Autodesk Inventor part; units mm, degrees
ref_plane "YZ Plane" through (0, 0, 0) normal (1, 0, 0) x (0, 1, 0)
ref_plane "XZ Plane" through (0, 0, 0) normal (0, 1, 0) x (-1, 0, 0)
ref_plane "XY Plane" through (0, 0, 0) normal (0, 0, 1) x (1, 0, 0)
sketch "스케치1" plane through (0, 0, 0) normal (0, 1, 0) x (-1, 0, 0)
  circle A0 centre (7.6948, -23.9851) radius 1.45
  circle A1 centre (27.7948, -23.9851) radius 1.45
  line L0 (-2.3552, -20.9851) -> (37.8448, -20.9851)
  line L1 (-2.3552, -20.9851) -> (-2.3552, -26.9851)
  line L2 (37.8448, -26.9851) -> (-2.3552, -26.9851)
  line L3 (37.8448, -20.9851) -> (37.8448, -26.9851)
  circle A2 centre (27.7948, 62.4149) radius 1.45
  circle A3 centre (7.6948, 62.4149) radius 1.45
  line L4 (37.8448, 65.4149) -> (-2.3552, 65.4149)
  line L5 (-2.3552, 65.4149) -> (-2.3552, 59.4149)
  line L6 (37.8448, 59.4149) -> (-2.3552, 59.4149)
  line L7 (37.8448, 65.4149) -> (37.8448, 59.4149)
  line L8 (37.8448, -20.9851) -> (-2.3552, -20.9851)
  line L9 (-2.3552, -20.9851) -> (-2.3552, 59.4149)
  line L10 (-2.3552, 59.4149) -> (37.8448, 59.4149)
  line L11 (37.8448, 59.4149) -> (37.8448, -20.9851)
  point P0 (0, 0)
extrude "돌출1" add sketch "스케치1" along normal blind 6 contours L9 L6 L11 L0
sketch "스케치2" plane through (0, 6, 0) normal (0, 1, 0) x (1, 0, 0)
  line L0 (2.3552, 20.9851) -> (-37.8448, 20.9851)
  line L1 (-37.8448, 20.9851) -> (-37.8448, -59.4149)
  line L2 (-37.8448, -59.4149) -> (2.3552, -59.4149)
  line L3 (2.3552, -59.4149) -> (2.3552, 20.9851)
  line L4 (-47.7448, 30.7851) -> (12.2552, -69.2149) construction
  line L5 (12.2552, 30.7851) -> (-47.7448, -69.2149) construction
  circle A0 centre (-7.6948, -39.3149) radius 1.35
  circle A1 centre (-27.7948, -39.3149) radius 1.35
  circle A2 centre (-7.6948, 0.8851) radius 1.35
  circle A3 centre (-27.7948, 0.8851) radius 1.35
  point P0 (0, 0)
  dimension "d2" = 60
  dimension "d3" = 100
  dimension "d4" = 2.7
  dimension "d5" = 2.7
  dimension "d6" = 2.7
  dimension "d27" = 2.7
extrude "돌출2" cut sketch "스케치2" against normal blind 6 contours A0 | A1 | A2 | A3
sketch "스케치3" plane through (-37.8448, 0, 59.4149) normal (0, 0, 1) x (1, 0, 0)
  line L0 (0, 0) -> (40.2, 0)
  line L1 (40.2, 0) -> (40.2, 6)
  line L2 (0, 6) -> (40.2, 6)
  line L3 (0, 0) -> (0, 6)
  line L4 (0, 6) -> (10.05, 6)
  line L5 (10.05, 6) -> (30.15, 6)
  circle A0 centre (10.05, 3) radius 1.35
  circle A1 centre (30.15, 3) radius 1.35
  point P0 (37.8448, 0)
  dimension "d9" = 40.2
  dimension "d10" = 6
  dimension "d11" = 10.05
  dimension "d12" = 20.1
  dimension "d13" = 2.7
  dimension "d14" = 2.7
extrude "돌출3" cut sketch "스케치3" against normal blind 16 contours A0 | A1
sketch "스케치4" plane through (2.3552, 0, -20.9851) normal (0, 0, -1) x (-1, 0, 0)
  circle A0 centre (30.15, 3) radius 1.35
  line L0 (11.4, 6) -> (11.4, 0)
  circle A1 centre (10.05, 3) radius 1.35
  point P0 (2.3552, 0)
extrude "돌출4" cut sketch "스케치4" against normal blind 16
sketch "스케치5" plane through (0, 6, 0) normal (0, 1, 0) x (1, 0, 0)
  line L0 (-29.1448, 20.9851) -> (-29.1448, 4.9851)
  line L1 (-26.4448, 20.9851) -> (-26.4448, 4.9851)
  line L2 (-29.1448, 4.9851) -> (-26.4448, 4.9851)
  line L3 (-9.0448, 20.9851) -> (-9.0448, 4.9851)
  line L4 (-6.3448, 20.9851) -> (-6.3448, 4.9851)
  line L5 (-9.0448, 4.9851) -> (-6.3448, 4.9851)
  circle A0 centre (-7.6948, 0.8851) radius 1.35
  circle A1 centre (-27.7948, 0.8851) radius 1.35
  circle A2 centre (-7.6948, -39.3149) radius 1.35
  circle A3 centre (-27.7948, -39.3149) radius 1.35
  line L6 (2.3552, 20.9851) -> (-37.8448, 20.9851)
  line L7 (-37.8448, 20.9851) -> (-37.8448, -59.4149)
  line L8 (-37.8448, -59.4149) -> (2.3552, -59.4149)
  line L9 (2.3552, -59.4149) -> (2.3552, 20.9851)
  line L10 (-9.0448, -59.4149) -> (-9.0448, -43.4149)
  line L11 (-29.1448, -59.4149) -> (-29.1448, -43.4149)
  line L12 (-26.4448, -59.4149) -> (-26.4448, -43.4149)
  line L13 (-6.3448, -59.4149) -> (-6.3448, -43.4149)
  line L14 (-30.3948, -52.5149) -> (-25.1948, -52.5149)
  line L15 (-25.1948, -52.5149) -> (-25.1948, -50.3149)
  line L16 (-25.1948, -50.3149) -> (-30.3948, -50.3149)
  line L17 (-30.3948, -50.3149) -> (-30.3948, -52.5149)
  line L18 (-30.3948, -52.5149) -> (-25.1948, -50.3149) construction
  line L19 (-25.1948, -52.5149) -> (-30.3948, -50.3149) construction
  line L20 (-10.2948, -52.5149) -> (-5.0948, -52.5149)
  line L21 (-5.0948, -52.5149) -> (-5.0948, -50.3149)
  line L22 (-5.0948, -50.3149) -> (-10.2948, -50.3149)
  line L23 (-10.2948, -50.3149) -> (-10.2948, -52.5149)
  line L24 (-10.2948, -52.5149) -> (-5.0948, -50.3149) construction
  line L25 (-5.0948, -52.5149) -> (-10.2948, -50.3149) construction
  line L26 (-30.3948, 11.8851) -> (-25.1948, 11.8851)
  line L27 (-25.1948, 11.8851) -> (-25.1948, 14.0851)
  line L28 (-25.1948, 14.0851) -> (-30.3948, 14.0851)
  line L29 (-30.3948, 14.0851) -> (-30.3948, 11.8851)
  line L30 (-30.3948, 11.8851) -> (-25.1948, 14.0851) construction
  line L31 (-25.1948, 11.8851) -> (-30.3948, 14.0851) construction
  line L32 (-10.2948, 11.8851) -> (-5.0948, 11.8851)
  line L33 (-5.0948, 11.8851) -> (-5.0948, 14.0851)
  line L34 (-5.0948, 14.0851) -> (-10.2948, 14.0851)
  line L35 (-10.2948, 14.0851) -> (-10.2948, 11.8851)
  line L36 (-10.2948, 11.8851) -> (-5.0948, 14.0851) construction
  line L37 (-5.0948, 11.8851) -> (-10.2948, 14.0851) construction
  point P0 (0, 0)
  point P1 (-27.7948, -51.4149)
  point P2 (-7.6948, -51.4149)
  point P3 (-27.7948, 12.9851)
  point P4 (-7.6948, 12.9851)
  dimension "d34" = 5.2
  dimension "d35" = 2.2
  dimension "d36" = 5.2
  dimension "d37" = 2.2
  dimension "d38" = 5.2
  dimension "d39" = 2.2
  dimension "d40" = 5.2
  dimension "d41" = 2.2
extrude "돌출5" cut sketch "스케치5" against normal blind 6 contours L28 L1 L26 L0 | L0 L26 L29 L28 | L28 L27 L26 L1 | L34 L4 L32 L3 | L3 L32 L35 L34 | L34 L33 L32 L4 | L14 L17 L16 L11 | L11 L16 L12 L14 | L12 L16 L15 L14 | L20 L23 L22 L10 | L10 L22 L13 L20 | L13 L22 L21 L20
sketch "스케치6" plane through (-37.8448, 0, 59.4149) normal (0, 0, 1) x (1, 0, 0)
  circle A0 centre (30.15, 3) radius 1.35
  circle A1 centre (10.05, 3) radius 1.35
  line L0 (0, 0) -> (40.2, 0)
  line L1 (40.2, 0) -> (40.2, 6)
  line L2 (0, 6) -> (40.2, 6)
  line L3 (0, 0) -> (0, 6)
  line L4 (15.1, 0) -> (25.1, 0)
  line L5 (25.1, 0) -> (25.1, 6)
  line L6 (25.1, 6) -> (15.1, 6)
  line L7 (15.1, 6) -> (15.1, 0)
  line L8 (15.1, 0) -> (25.1, 6) construction
  line L9 (25.1, 0) -> (15.1, 6) construction
  point P0 (37.8448, 0)
  point P1 (20.1, 3)
  dimension "d28" = 10
extrude "돌출6" add sketch "스케치6" along normal blind 6 contours L7 L2 L5 L0
sketch "스케치7" plane through (2.3552, 0, -20.9851) normal (0, 0, -1) x (-1, 0, 0)
  line L0 (15.1, 6) -> (15.1, 0)
  line L1 (25.1, 0) -> (25.1, 6)
  circle A0 centre (30.15, 3) radius 1.35
  circle A1 centre (10.05, 3) radius 1.35
  line L2 (0, 0) -> (40.2, 0)
  line L3 (40.2, 0) -> (40.2, 6)
  line L4 (0, 6) -> (40.2, 6)
  line L5 (0, 0) -> (0, 6)
  point P0 (2.3552, 0)
extrude "돌출7" add sketch "스케치7" along normal blind 6 contours L4 L1 L2 L0
properties part number "feet_holder3" material "PMMA 플라스틱"
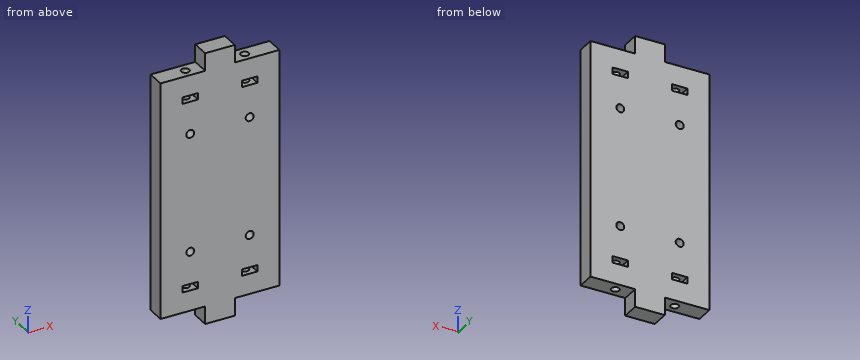
Source: CAD feature listing. Evaluate the final solid. Frame: model axes, mm. Coordinates: 2 decimals unless noted, no trailing zeros. Write each loop counter-clockwise with the first axis right and the second up, starting at its lowest first coordinate (ties: lowest second). Pieces come first, ordered by that corner, then holes. Notation, with made-up numbers: (-10, 68) -> (-4, 68) arc R28 ccw to (-4, 100) -> close; hole circle Ø11 at (89.5, -21). An arc over 180 degrees is marked (long way). Return JSON: item names as keys, results as strings. Group by question number.
1) Section query A-A, the plane z = -13. Return loops of the section in (x, y), plus the area to 3 significant figures.
2) Ray query, line 1 along Z through (x, y) = (-9.5, 4.2); line 2 along X through (y, z) = (3.1, 52); line 3 along X through (y, z) = (5.05, 61). Return the intervals inside material, ascending.
3) Section query C-C, the plane y = 3. State how many separate pieces and enclosed holes the cut face has, plus the area to 3 significant figures.
4) Contact query for flat-ended pins moving along their axis: P1, Ø1.6, axis at x = -27.79, y = 3, coming from the +Z side; P2, Ø3.5, axis at x = -7.69, y = 3, coming from the +Z side; P3, Ø2, axis at x = -7.69, y = 3, coming from the -Z side; P4, Ø1.6, axis at x = -27.79, z = -0.89, coming from the -Y side. Output: stop coordinate, or through.
5) Section query B-B, the plane x = 0.5. Return loops of the section in (y, z), plus the area to 3 significant figures.
From the geometry:
{
 "1": {"outline": "(-37.84, 0) -> (-30.39, 0) -> (-30.39, 6) -> (-37.84, 6) -> close; (-25.19, 0) -> (-10.29, 0) -> (-10.29, 6) -> (-25.19, 6) -> close; (-5.09, 0) -> (2.36, 0) -> (2.36, 6) -> (-5.09, 6) -> close", "area": "179 mm²"},
 "2": {"line 1": "-20.99 to -14.09, -11.89 to 50.31, 52.51 to 59.41", "line 2": "-37.84 to -30.39, -25.19 to -10.29, -5.09 to 2.36", "line 3": "-22.74 to -12.74"},
 "3": {"separate pieces": "1", "enclosed holes": "4", "area": "3,130 mm²"},
 "4": {"P1": "z = 43.41", "P2": "z = 59.41", "P3": "z = -4.99", "P4": "through"},
 "5": {"outline": "(0, -20.99) -> (6, -20.99) -> (6, 59.41) -> (0, 59.41) -> close", "area": "482 mm²"}
}
